The figure shows three views and two pictorial views of one solid part (mm, origin at its lowest corner). Answer the questions. Coordinates: 2 decimals unless noted, no trailing zeros. Order: outer loops, then holes, each group sorted by start corner. A loop starts at its lowest first (then second) coordinate and runs counter-clockwise, first axis right, second up.
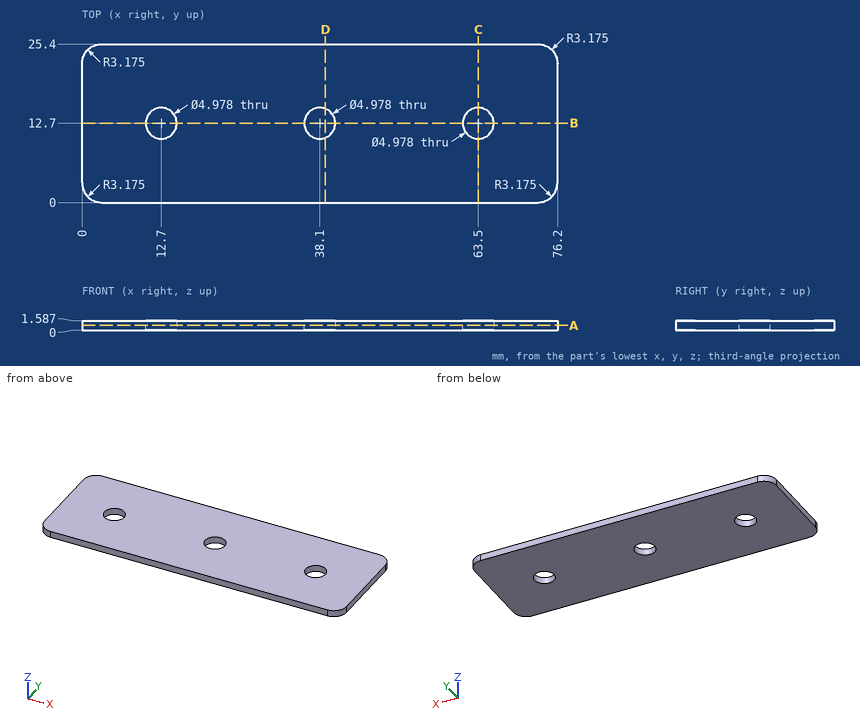
Q1. The part is cut by section B-B, the plane y = 12.7. Determine the outline of the cut face in (x, z).
Q2. The part is cut by section C-C, the plane x = 63.5. Determine the outline of the cut face in (y, z).
Q3. The part is cut by section D-D, the plane x = 39. Determine the outline of the cut face in (y, z).
Q4. Straight lines are drawn through the part: L1, parallel to Y at x = 38.1, z = 1.2; L2, parallel to Y at x = 39, z = 0.1; L3, parallel to X at y = 1.5, z = 1.25. For each, find the intervals that lie inside material, in ascending order.
Q5. The part is cut by section A-A, the plane z = 0.8. State how many separate pieces and enclosed holes the cut face has, then the cut area to 3 significant figures.
Q6. Each of these flat-tipped pins is pushed along its axis until it touches: P1, Ø10, axis at x = 68.5, y = 8.5, coming from the -Z side; P2, Ø4, axis at x = 12.7, y = 12.7, coming from the +Z side (1 decimal). Where does it stop, or does it pass through?
Computed values:
1. outline: (0, 0) - (10.21, 0) - (10.21, 1.59) - (0, 1.59) - close; (15.19, 0) - (35.61, 0) - (35.61, 1.59) - (15.19, 1.59) - close; (40.59, 0) - (61.01, 0) - (61.01, 1.59) - (40.59, 1.59) - close; (65.99, 0) - (76.2, 0) - (76.2, 1.59) - (65.99, 1.59) - close
2. outline: (0, 0) - (10.21, 0) - (10.21, 1.59) - (0, 1.59) - close; (15.19, 0) - (25.4, 0) - (25.4, 1.59) - (15.19, 1.59) - close
3. outline: (0, 0) - (10.38, 0) - (10.38, 1.59) - (0, 1.59) - close; (15.02, 0) - (25.4, 0) - (25.4, 1.59) - (15.02, 1.59) - close
4. L1: y = 0 to 10.21, 15.19 to 25.4
4. L2: y = 0 to 10.38, 15.02 to 25.4
4. L3: x = 0.48 to 75.72
5. separate pieces: 1
5. enclosed holes: 3
5. area: 1,870 mm2
6. P1: stops at z = 0
6. P2: passes through
